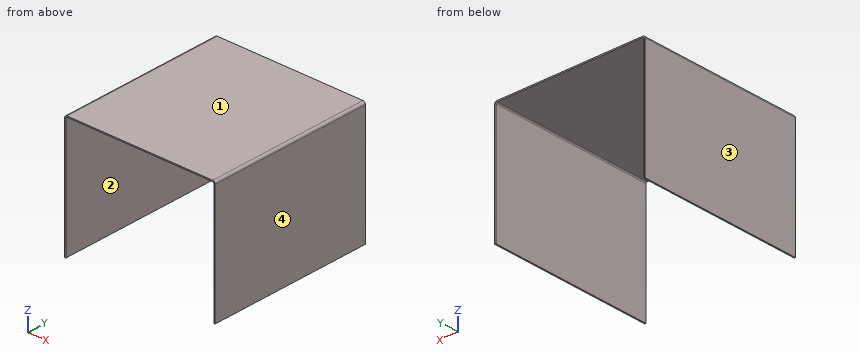
Autodesk Inventor part; units mm, degrees
ref_plane "YZ Plane" through (0, 0, 0) normal (1, 0, 0) x (0, 1, 0)
ref_plane "XZ Plane" through (0, 0, 0) normal (0, 1, 0) x (-1, 0, 0)
ref_plane "XY Plane" through (0, 0, 0) normal (0, 0, 1) x (1, 0, 0)
sketch "Sketch1" plane through (0, 0, 0) normal (0, 0, 1) x (1, 0, 0)
  line L0 (125, -136.782) -> (-125, -136.782)
  line L1 (-125, -136.782) -> (-125, 136.782)
  line L2 (-125, 136.782) -> (125, 136.782)
  line L3 (125, 136.782) -> (125, -136.782)
  line L4 (125, -136.782) -> (-125, 136.782) construction
  line L5 (-125, -136.782) -> (125, 136.782) construction
  point P0 (0, 0)
  dimension "d1" = 250
extrude "Plate1" add sketch "Sketch1" along normal blind 2
sketch "Sketch2" plane through (123, -136.782, 2) normal (1, 0, 0) x (0, 1, 0)
  line L0 (273.5641, 0) -> (0, 0)
  line L1 (0, 0) -> (0, -200)
  line L2 (0, -200) -> (273.5641, -200)
  line L3 (273.5641, -200) -> (273.5641, 0)
edge flange "Flange1" height 200 angle 90 thickness 2 bend radius 2 thickness toward (1, 0, 0) relief tear relief width 2 relief depth 1 edges at (125, 0, 0) wall of the first edge with corners at (123, 136.782, 2) (123, -136.782, 2) (123, -136.782, -198) (123, 136.782, -198)
bend "Bend1"
corner "Corner1"
sketch "Sketch3" plane through (-123, 136.782, 2) normal (-1, 0, 0) x (0, -1, 0)
  line L0 (273.5641, 0) -> (0, 0)
  line L1 (0, 0) -> (0, -200)
  line L2 (0, -200) -> (273.5641, -200)
  line L3 (273.5641, -200) -> (273.5641, 0)
edge flange "Flange2" height 200 angle 90 thickness 2 bend radius 2 thickness toward (-1, 0, 0) relief tear relief width 2 relief depth 1 edges at (-125, 0, 0) wall of the first edge with corners at (-123, -136.782, 2) (-123, 136.782, 2) (-123, 136.782, -198) (-123, -136.782, -198)
bend "Bend2"
corner "Corner2"
equation "\"d0\" = Thickness"
equation "\"d2\" = BendReliefWidth"
equation "\"d3\" = BendReliefDepth"
equation "\"d4\" = MinimumRemnant"
equation "\"d5\" = TransitionRadius"
equation "\"d8\" = BendRadius"
equation "\"d9\" = CornerReliefSize"
equation "\"d10\" = GapSize"
equation "\"d11\" = JacobiRadiusSize"
equation "\"d12\" = BendReliefWidth"
equation "\"d13\" = BendReliefDepth"
equation "\"d14\" = MinimumRemnant"
equation "\"d15\" = TransitionRadius"
equation "\"d18\" = BendRadius"
equation "\"d19\" = CornerReliefSize"
equation "\"d20\" = GapSize"
equation "\"d21\" = JacobiRadiusSize"
equation "\"BendRadius\" = Thickness"
equation "\"BendReliefWidth\" = Thickness"
equation "\"BendReliefDepth\" = 0.5 * Thickness"
equation "\"CornerReliefSize\" = 4 * Thickness"
equation "\"MinimumRemnant\" = 2 * Thickness"
equation "\"TransitionRadius\" = BendRadius"
equation "\"JacobiRadiusSize\" = BendRadius"
equation "\"GapSize\" = Thickness"
Read the model definition and answer for the solid it produces. Units are mm, in the model's axes. Face numbers are marked on the shaded views. Coordinates: 2 decimals unless noted, no trailing zeros. Order: outer loops, then holes, each group sorted by start corner. A loop starts at its lowest first (then second) coordinate and runs counter-clockwise, first axis right, second up. Notation, with made-up numbers: (-11.5, 53.5) - (46.5, 53.5) arc R15 cw to (46.5, 66.5) - close; hole circle Ø4 at (88, -1.5). An arc over 180 degrees is marked (long way). Answer as a JSON object with one key per item and string values. Group by question number.
Item 1: Section A-A (z = -27) is taken. Give the vertices of the cut face in (x, y).
Item 2: Section B-B (y = -9) is taken. Give the vertices of the cut face in (x, z), plus the area to 3 significant figures.
Item 3: Section C-C (x = 63) is taken. Give the vertices of the cut face in (y, z).
Item 4: Consider probe 1 along X at (y, z) = (14, -149); probe 2 along Z at (x, y) = (98, 14.5). Determine where each line is inside the solid, lowest interval first. Write a range as from..to.
Item 5: A flat-ended cylindrical pin translates along its axis: P1, Ø6, axis at x = 83, y = 39, coming from the -Z side. Find the tip coordinate at first contact, or state that the pin passes through.
Item 6: The mould has two halves that part along X. Classify the marked faces 1, 2, 3 and 4: +X half, -X half, draft (parallel to the pull), parting line (faces both ways), or undercut.
Results are:
{
 "1": {"outline": "(-125, -136.78) - (-123, -136.78) - (-123, 136.78) - (-125, 136.78) - close; (123, -136.78) - (125, -136.78) - (125, 136.78) - (123, 136.78) - close"},
 "2": {"outline": "(-125, -198) - (-123, -198) - (-123, -2) arc R2 cw to (-121, 0) - (121, 0) arc R2 cw to (123, -2) - (123, -198) - (125, -198) - (125, -2) arc R4 ccw to (121, 2) - (-121, 2) arc R4 ccw to (-125, -2) - close", "area": "1,290 mm^2"},
 "3": {"outline": "(-136.78, 0) - (136.78, 0) - (136.78, 2) - (-136.78, 2) - close"},
 "4": {"probe 1": "x = -125..-123, 123..125", "probe 2": "z = 0..2"},
 "5": {"P1": "stops at z = 0"},
 "6": {"face 1": "draft", "face 2": "undercut", "face 3": "-X half", "face 4": "+X half"}
}
